from build123d import *


with BuildPart() as part:
    # Sketch → Revolution (revolve)
    with BuildSketch(Plane.XZ):
        Polygon((0, 0), (20.75, 0), (20.75, 5), (18.75, 5), (18.75, 1), (11.35, 1), (11.35, 5), (9.35, 5), (9.35, 1), (0, 1), align=None)
    revolve(axis=Axis((0, 0, 0), (0, 0, 1)))


solid = part.part
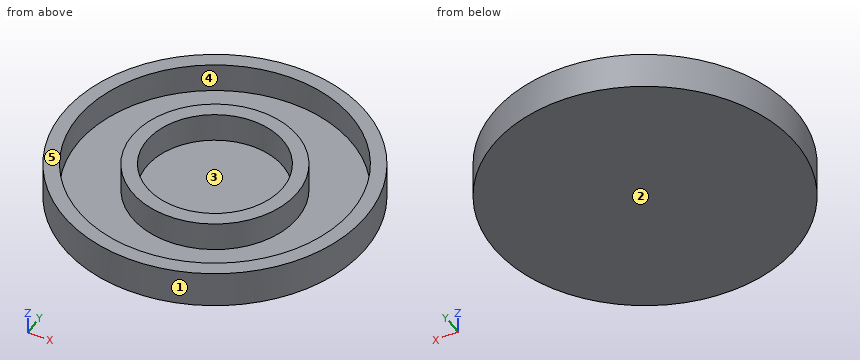
The model under review builds one solid part; all positions refer to its coordinate system, in mm. Face numbers are marked on the shaded views. A direction names the side the tool comes from. Round coordinates to 2 decimals unless told otherwise and drop trailing zeros. Write each loop counter-clockwise with the first axis right and the second up, starting at its lowest first coordinate (ties: lowest second). Pieces come first, ordered by that corner, then holes. Notation, with made-up numbers: M 79.25,-20.5 L 111.25,-20.5 A16 cw 111.25,-1.5 Z; hole C -14.75,68 d10. An arc over 180 degrees is marked long. Use a Markdown table: item, result. Add a question column.
Q1. To check wall thickness, follow line 1 (Y direction, x = 0, z = 2.3); line 2 (Z direction, x = -16, y = -9); line 3 (X direction, y = 12.5, z = 4.1). State the ranges of each line that lie inside material, in increasing order.
Q2. Machinability: for the marked faces 4 and 5, which of the approach directions +Z, -Z, +X, -X, +Y, -Y give a long, thin tool a straight path to every point of the face, cutting with its end or side? Answer none if there is none.
Q3. We need section B-B, the plane z = 1.75. State the section outline as (x, y) points, plus the area to 3 significant figures.
Q4. We need section D-D, the plane x = 18. State the section outline as (y, z) points, plus the area to 3 significant figures.
Q5. We need section A-A, the plane y = 0. State the section outline as (x, z) points, plus the area to 3 significant figures.
Q6. Insertion check: pin 1 (5.5 mm diameter, centred on x = 2, y = 4.5, fed in from +Z); pin 2 (3 mm diameter, centred on y = 8, z = 0.5, fed in from +X); pin 3 (1.5 mm diameter, centred on x = -5.5, z = 0.5, fed in from -Y). Each pin has a flat end and moves straight along its axis. Give the tip position at first contact, or say it passes through.
Q7. The part is to be moulded in two halves that separate along X. For the marked faces 1, 2 and 3, say which applies: pulls with the +X half, pulls with the -X half, needs draft (parallel to the pull), parting line crosses it, or undercut.
Findings below:
| question | item | result |
|---|---|---|
| 1 | line 1 | y = -20.75 to -18.75, -11.35 to -9.35, 9.35 to 11.35, 18.75 to 20.75 |
| 1 | line 2 | z = 0 to 1 |
| 1 | line 3 | x = -16.56 to -13.98, 13.98 to 16.56 |
| 2 | face 4 | +Z |
| 2 | face 5 | +Z, +X, -X, +Y, -Y |
| 3 | outline | C 0,0 d41.5; C 0,0 d22.7; hole C 0,0 d37.5; hole C 0,0 d18.7 |
| 3 | area | 378 mm² |
| 4 | outline | M -10.32,0 L 10.32,0 L 10.32,5 L 5.25,5 L 5.25,1 L -5.25,1 L -5.25,5 L -10.32,5 Z |
| 4 | area | 61.2 mm² |
| 5 | outline | M -20.75,0 L 20.75,0 L 20.75,5 L 18.75,5 L 18.75,1 L 11.35,1 L 11.35,5 L 9.35,5 L 9.35,1 L -9.35,1 L -9.35,5 L -11.35,5 L -11.35,1 L -18.75,1 L -18.75,5 L -20.75,5 Z |
| 5 | area | 73.5 mm² |
| 6 | pin 1 | stops at z = 1 |
| 6 | pin 2 | stops at x = 19.71 |
| 6 | pin 3 | stops at y = -20.2 |
| 7 | face 1 | parting line crosses it |
| 7 | face 2 | needs draft |
| 7 | face 3 | undercut |
